from build123d import *

# Parameters (mm, degrees)
F1_DEPTH      = 20
F1_DEPTH_BACK = 20
F2_R          = 10
F3_DEPTH      = 3
F4_R          = 10
F5_DEPTH      = 3


with BuildPart() as f1:
    # F0 (on Front) → F1 (new body, two sides)
    with BuildSketch(Plane.XZ) as f1_sk:
        with BuildLine():
            ThreePointArc((4, -4.472136), (-6, 0), (4, 4.472136))
            Line((4, 4.472136), (4, 20))
            Line((4, 20), (-23, 20))
            Line((-23, 20), (-23, -20))
            Line((-23, -20), (4, -20))
            Line((4, -20), (4, -4.472136))
        make_face()
    extrude(amount=F1_DEPTH)
    extrude(f1_sk.sketch, amount=-F1_DEPTH_BACK)

    # F2 (on face) → F3 (cut)
    with BuildSketch(Plane(origin=(0, 20, 0), x_dir=(-1, 0, 0), z_dir=(0, 1, 0))):
        Circle(F2_R)
    extrude(amount=-F3_DEPTH, mode=Mode.SUBTRACT)

    # F4 (on face) → F5 (cut)
    with BuildSketch(Plane.XZ.offset(20)):
        Circle(F4_R)
    extrude(amount=-F5_DEPTH, mode=Mode.SUBTRACT)


solid = f1.part
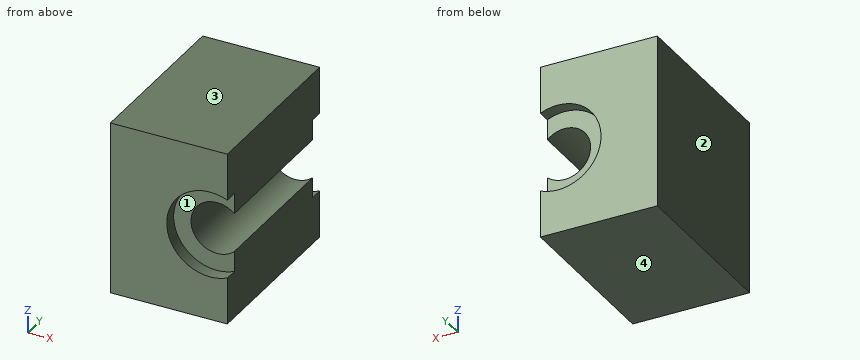
Geometry check sheet. Reference: the model listing, model coordinates, mm. Face numbers are marked on the shaded views. Give positions to 0.01 mm unless a question says otherwise; leave off trailing zeros. Write each loop counter-clockwise with the first axis right and the second up, starting at its lowest first coordinate (ties: lowest second). Pieces come first, ordered by that corner, then holes. Notation, with made-up numbers: (51, 16.25) - (109, 16.25) arc R17 ccw to (109, 23.25) - close; hole circle Ø3 at (-23.75, 76). An arc over 180 degrees is marked (long way). Put each result on its own line as item: value.
1. Sectioned sample at D-D, the plane x = -9. Enter the section's corners in (y, z).
Ans:
outline: (-20, -20) - (20, -20) - (20, -4.36) - (17, -4.36) - (17, 4.36) - (20, 4.36) - (20, 20) - (-20, 20) - (-20, 4.36) - (-17, 4.36) - (-17, -4.36) - (-20, -4.36) - close
2. Thickness scan on line 1 (Z direction, x = 0, y = 1); line 2 (Z direction, x = 0, y = -19.1); line 3 (Y direction, x = -9, z = -3.5). Record the ranges inside material, lowest first.
Ans:
line 1: z = -20 to -6, 6 to 20
line 2: z = -20 to -10, 10 to 20
line 3: y = -17 to 17
3. Go/stop test with flat-tipped pins: pin 1 (16 mm diameter, centred on x = 0, z = 0, fed in from -Y); pin 2 (15.5 mm diameter, centred on x = 0, z = -0.5, fed in from +Y). Record where each tip stops, or that it passes through.
Ans:
pin 1: stops at y = -17
pin 2: stops at y = 17
4. Sectioned sample at A-A, the plane x = 0. Enter the section's corners in (y, z), plus the area to 3 significant figures.
Ans:
outline: (-20, -20) - (20, -20) - (20, -10) - (17, -10) - (17, -6) - (-17, -6) - (-17, -10) - (-20, -10) - close; (-20, 10) - (-17, 10) - (-17, 6) - (17, 6) - (17, 10) - (20, 10) - (20, 20) - (-20, 20) - close
area: 1,070 mm²
5. Draft check along Z on the marked faces 1, 2, 3 and 4. Enter one of: +Z half, -Z half, draft (parallel to the pull), parting line (faces both ways), or undercut.
Ans:
face 1: undercut
face 2: draft
face 3: +Z half
face 4: -Z half
6. Sectioned sample at B-B, the plane z = -8. Enter the section's corners in (x, y), plus the area to 3 significant figures.
Ans:
outline: (-23, -20) - (-6, -20) - (-6, -17) - (4, -17) - (4, 17) - (-6, 17) - (-6, 20) - (-23, 20) - close
area: 1,020 mm²
7. Sectioned sample at C-C, the plane y = -2. Enter the section's corners in (x, z), plus the area to 3 significant figures.
Ans:
outline: (-23, -20) - (4, -20) - (4, -4.47) arc R6 cw (long way) to (4, 4.47) - (4, 20) - (-23, 20) - close
area: 979 mm²
